Design review of the part built by this model. Coordinates are the model's own, in mm. Face numbers are marked on the shaded views. A direction names the side the tool comes from. Round coordinates to 2 decimals unless told otherwise and drop trailing zeros. Loops run counter-clockwise (first coordinate to the right, second up) from the corner with the lowest first, then second, coordinate; pieces in that order, holes last. Notation, with made-up numbers: (-9, 71.25) - (37, 71.25) arc R22 ccw to (37, 106.25) - close; hole circle Ø9 at (-21, 36.25). An arc over 180 degrees is marked (long way). Answer as CSV lines item,"result". Start each with the question number.
(1) Consider section D-D (z = 26.5). Give the boundary of the cut face in (x, y).
(2) For the marked faces 1, 2 and 3, list the 3-axis set-ups (+Z, -Z, +X, -X, +Y, -Y) from which the entire face can be reached by the end or side of a thin tool; tool diameter is ignored.
(3) Wall thickness on L1, parallel to X at y = 3.85, z = 0; L2, parallel to Y at x = -28, z = 12.5; L3, parallel to Z at x = -33.5, y = -31.5: over which ranges is each line inside the solid? List them lowest first.
(4) Mouldability with a two-part tool opening along X and no side actions: class the marked faces 4, 5, 6 and 7 as released by +X, released by -X, zero draft, split by the parting line, or undercut.
(5) Consider section C-C (z = 0). Give the boundary of the cut face in (x, y).
(6) Consider section B-B (y = -17). Count the separate pieces of the cut face and the enclosed holes in it, and give its area (3 significant figures).
(7) Consider section A-A (x = -30). Give the boundary of the cut face in (y, z).
(8) For P1, Ø12, axis at x = 26, y = -5.5, coming from the +Z side; P2, Ø6, axis at x = 30, z = 0, coming from the +Y side; P3, Ø1.6, axis at x = 5, y = -1.5, coming from the -Z side, all flat-tipped, find the tip position at first contact; note any pin that passes through.
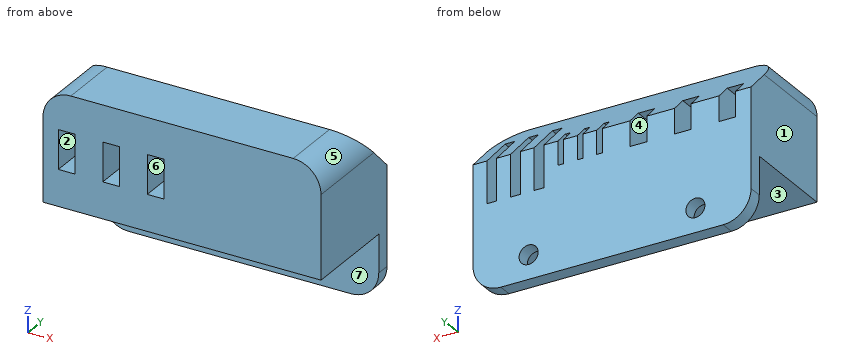
from build123d import *

# Parameters (mm, degrees)
SKETCH1_W           = 100
SKETCH1_H           = 30
BOSS_EXTRUDE1_DEPTH = 5
SKETCH2_W           = 100
SKETCH2_H           = 40
BOSS_EXTRUDE2_DEPTH = 40
SKETCH3_W           = 3.5
SKETCH3_H           = 26
CUT_EXTRUDE1_DEPTH  = 25
SKETCH4_W           = 2
SKETCH4_H           = 13
CUT_EXTRUDE2_DEPTH  = 10
SKETCH5_W           = 6
SKETCH5_H           = 14
CUT_EXTRUDE3_DEPTH  = 85.409715081
CHAMFER1_SIZE       = 18
SKETCH6_R           = 3.429
CUT_EXTRUDE4_DEPTH  = 85.409715081
SKETCH7_W           = 100
SKETCH7_H           = 6.35
CUT_EXTRUDE5_DEPTH  = 85.409715081
FILLET1_R           = 10


with BuildPart() as part:
    # Sketch1 → Boss-Extrude1 (new body)
    with BuildSketch(Plane(origin=(0, 0, 0), x_dir=(1, 0, 0), z_dir=(0, 1, 0))):
        Rectangle(SKETCH1_W, SKETCH1_H)
    extrude(amount=BOSS_EXTRUDE1_DEPTH)

    # Sketch2 → Boss-Extrude2 (add)
    with BuildSketch(Plane.XY.offset(15)):
        with Locations((0, -15)):
            Rectangle(SKETCH2_W, SKETCH2_H)
    extrude(amount=BOSS_EXTRUDE2_DEPTH)

    # Sketch3 → Cut-Extrude1 (cut)
    with BuildSketch(Plane(origin=(0, 5, 0), x_dir=(1, 0, 0), z_dir=(0, 1, 0))):
        with Locations((43.25, -35)):
            Rectangle(SKETCH3_W, SKETCH3_H)
        with Locations((34.75, -35)):
            Rectangle(SKETCH3_W, SKETCH3_H)
        with Locations((26.25, -35)):
            Rectangle(SKETCH3_W, SKETCH3_H)
    extrude(amount=-CUT_EXTRUDE1_DEPTH, mode=Mode.SUBTRACT)

    # Sketch4 → Cut-Extrude2 (cut)
    with BuildSketch(Plane(origin=(0, 5, 0), x_dir=(1, 0, 0), z_dir=(0, 1, 0))):
        with Locations((18.5, -35)):
            Rectangle(SKETCH4_W, SKETCH4_H)
        with Locations((11.5, -35)):
            Rectangle(SKETCH4_W, SKETCH4_H)
        with Locations((4.5, -35)):
            Rectangle(SKETCH4_W, SKETCH4_H)
    extrude(amount=-CUT_EXTRUDE2_DEPTH, mode=Mode.SUBTRACT)

    # Sketch5 → Cut-Extrude3 (cut, through all)
    with BuildSketch(Plane(origin=(0, 5, 0), x_dir=(1, 0, 0), z_dir=(0, 1, 0))):
        with Locations((-9.5, -35)):
            Rectangle(SKETCH5_W, SKETCH5_H)
        with Locations((-25.5, -35)):
            Rectangle(SKETCH5_W, SKETCH5_H)
        with Locations((-41.5, -35)):
            Rectangle(SKETCH5_W, SKETCH5_H)
    extrude(amount=-CUT_EXTRUDE3_DEPTH, mode=Mode.SUBTRACT)

    # Chamfer1
    # the kernel refuses this chamfer: 18 mm, written as the material it takes off along each edge
    with BuildSketch(Plane(origin=(-96.290293783, 5, 55), x_dir=(0, -0.9996219169112966, 0.02749587661058639), z_dir=(1, 0, 0))) as chamfer1_piece_1:
        Polygon((CHAMFER1_SIZE * 0.999621916911, CHAMFER1_SIZE * 0.0274958766106), (-CHAMFER1_SIZE * 0.0274958766106, CHAMFER1_SIZE * 0.999621916911), (0, 0), align=None)
    extrude(amount=192.580587567, mode=Mode.SUBTRACT)

    # Sketch6 → Cut-Extrude4 (cut, through all)
    with BuildSketch(Plane(origin=(0, 5, 0), x_dir=(1, 0, 0), z_dir=(0, 1, 0))):
        with Locations(Location((-30, 0, 0), (0, 0, 270))):
            Circle(SKETCH6_R)
        with Locations(Location((30, 0, 0), (0, 0, 270))):
            Circle(SKETCH6_R)
    extrude(amount=-CUT_EXTRUDE4_DEPTH, mode=Mode.SUBTRACT)

    # Sketch7 → Cut-Extrude5 (cut, through all)
    with BuildSketch(Plane(origin=(0, 5, 0), x_dir=(1, 0, 0), z_dir=(0, 1, 0))):
        with Locations((0, 11.825)):
            Rectangle(SKETCH7_W, SKETCH7_H)
    extrude(amount=-CUT_EXTRUDE5_DEPTH, mode=Mode.SUBTRACT)

    # Fillet1
    fillet1_edges = [part.edges().sort_by_distance(p)[0] for p in [
        (-50, -24, 55),
        (50, -24, 55),
        (-50, 2.5, -8.65),
        (50, 2.5, -8.65),
    ]]
    fillet(fillet1_edges, radius=FILLET1_R)


solid = part.part
Determined:
1,outline,"(-50, -35) - (50, -35) - (50, 5) - (45, 5) - (45, -20) - (41.5, -20) - (41.5, 5) - (36.5, 5) - (36.5, -20) - (33, -20) - (33, 5) - (28, 5) - (28, -20) - (24.5, -20) - (24.5, 5) - (-50, 5) - close"
2,face 1,"+Z, -Z, -X, +Y, -Y"
2,face 2,"+Y, -Y"
2,face 3,"-Z, +X, -X, -Y"
3,L1,"x = -49.91 to -33.43, -26.57 to 26.57, 33.43 to 49.91"
3,L2,"y = 0 to 5"
3,L3,"z = 15 to 55"
4,face 4,"undercut"
4,face 5,"released by +X"
4,face 6,"undercut"
4,face 7,"zero draft"
5,outline,"(-49.91, 0) - (-33.43, 0) - (-33.43, 5) - (-49.91, 5) - close; (-26.57, 0) - (26.57, 0) - (26.57, 5) - (-26.57, 5) - close; (33.43, 0) - (49.91, 0) - (49.91, 5) - (33.43, 5) - close"
6,separate pieces,"1"
6,enclosed holes,"6"
6,area,"3,430 mm^2"
7,outline,"(-35, 15) - (0, 15) - (0, 3.43) - (5, 3.43) - (5, 37) - (-13, 55) - (-35, 55) - close; (0, -8.65) - (5, -8.65) - (5, -3.43) - (0, -3.43) - close"
8,P1,"stops at z = 53.5"
8,P2,"passes through"
8,P3,"stops at z = 15"
